from build123d import *

# Parameters (mm, degrees)
CROQUIS1_W              = 700
CROQUIS1_H              = 700
CROQUIS1_W_2            = 600
CROQUIS1_H_2            = 600
SALIENTE_EXTRUIR1_DEPTH = 50
CROQUIS2_W              = 50
CROQUIS2_H              = 50
SALIENTE_EXTRUIR2_DEPTH = 1800
CROQUIS3_W              = 700
CROQUIS3_H              = 700
CROQUIS3_W_2            = 600
CROQUIS3_H_2            = 600
SALIENTE_EXTRUIR3_DEPTH = 50
CROQUIS4_W              = 700
CROQUIS4_H              = 700
CROQUIS4_W_2            = 600
CROQUIS4_H_2            = 600
SALIENTE_EXTRUIR4_DEPTH = 50
CROQUIS6_W              = 122.530736156
CROQUIS6_H              = 155
CROQUIS6_W_2            = 72.530736156
CROQUIS6_H_2            = 80
SALIENTE_EXTRUIR5_DEPTH = 50
CROQUIS7_W              = 25
CROQUIS7_H              = 25
SALIENTE_EXTRUIR6_DEPTH = 100
SALIENTE_EXTRUIR7_DEPTH = 15


with BuildPart() as part:
    # Croquis1 → Saliente-Extruir1 (new body)
    with BuildSketch(Plane(origin=(0, 0, 0), x_dir=(1, 0, 0), z_dir=(0, 1, 0))):
        with Locations((300, 300)):
            Rectangle(CROQUIS1_W, CROQUIS1_H)
        with Locations((300, 300)):
            Rectangle(CROQUIS1_W_2, CROQUIS1_H_2, mode=Mode.SUBTRACT)
    extrude(amount=SALIENTE_EXTRUIR1_DEPTH)

    # Croquis2 → Saliente-Extruir2 (add)
    with BuildSketch(Plane.XZ):
        with Locations((625, 25)):
            Rectangle(CROQUIS2_W, CROQUIS2_H)
        with Locations((-25, 25)):
            Rectangle(CROQUIS2_W, CROQUIS2_H)
        with Locations((-25, -625)):
            Rectangle(CROQUIS2_W, CROQUIS2_H)
        with Locations((625, -625)):
            Rectangle(CROQUIS2_W, CROQUIS2_H)
    extrude(amount=SALIENTE_EXTRUIR2_DEPTH)

    # Croquis3 → Saliente-Extruir3 (add)
    with BuildSketch(Plane(origin=(0, -725, 0), x_dir=(-1, 0, 0), z_dir=(0, -1, 0))):
        with Locations((-300, 300)):
            Rectangle(CROQUIS3_W, CROQUIS3_H)
        with Locations((-300, 300)):
            Rectangle(CROQUIS3_W_2, CROQUIS3_H_2, mode=Mode.SUBTRACT)
    extrude(amount=SALIENTE_EXTRUIR3_DEPTH)

    # Croquis4 → Saliente-Extruir4 (add)
    with BuildSketch(Plane(origin=(0, -50, 0), x_dir=(-1, 0, 0), z_dir=(0, -1, 0))):
        with Locations((-300, 300)):
            Rectangle(CROQUIS4_W, CROQUIS4_H)
        with Locations((-300, 300)):
            Rectangle(CROQUIS4_W_2, CROQUIS4_H_2, mode=Mode.SUBTRACT)
    extrude(amount=SALIENTE_EXTRUIR4_DEPTH)

    # Croquis6 → Saliente-Extruir5 (add)
    with BuildSketch(Plane.XY.offset(50)):
        with Locations((446.741550776, 77.5)):
            Rectangle(CROQUIS6_W, CROQUIS6_H)
        with Locations((446.741550776, 90)):
            Rectangle(CROQUIS6_W_2, CROQUIS6_H_2, mode=Mode.SUBTRACT)
    extrude(amount=-SALIENTE_EXTRUIR5_DEPTH)

    # Croquis7 → Saliente-Extruir6 (add)
    with BuildSketch(Plane(origin=(0, 0, 0), x_dir=(-1, 0, 0), z_dir=(0, 0, -1))):
        with Locations((-445.476182698, 142.5)):
            Rectangle(CROQUIS7_W, CROQUIS7_H)
    extrude(amount=SALIENTE_EXTRUIR6_DEPTH)

    # Croquis9 → Saliente-Extruir7 (add, symmetric)
    with BuildSketch(Plane.ZY.offset(-90)):
        Polygon((0, 50), (50, 50), (50, 290), (-650, 290), (-650, 50), (-600, 50), (-600, 240), (0, 240), align=None)
    extrude(amount=SALIENTE_EXTRUIR7_DEPTH, both=True)


solid = part.part
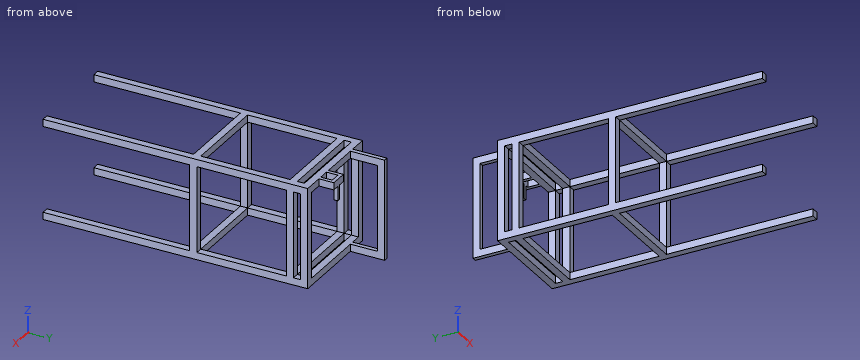
Model file for the job. Use its own axes, mm. Give positions to 0.01 mm unless a question says otherwise; leave off trailing zeros. Order: outer loops, then holes, each group sorted by start corner. A loop starts at its lowest first (then second) coordinate and runs counter-clockwise, first axis right, second up. Notation, with made-up numbers: M 43.25,30 L 75.25,30 A18 cw 75.25,44 Z; hole C -32.5,53 d8. An arc over 180 degrees is marked long. Put each result on its own line as item: value. Start each with the question number.
(1) Band-saw the part on A-A on x = 20. Give the cut face in (y, z).
(2) Drill centre lines: L1, parallel to Y at x = -13.5, z = -141; L2, parallel to Y at x = 472, z = 4; L3, parallel to X at y = -823.5, z = -608.5. Where is each one in solid material? Low to high. Write a range as [from, to].
(3) Band-saw the part on B-B on y = -300.5. Give the cut face in (x, z).
(4) Pin check, flat tips, straight feed: pin 1 Ø15 at (x, z) = (625.5, -358.5) entering from +Y; pin 2 Ø15 at (x, z) = (340.5, -631) entering from -Y. Stop position of each tip, or through.
(5) Band-saw the part on C-C on z = -259. Give the cut face in (x, y).
Results below:
1. outline: M -775,-650 L -725,-650 L -725,-600 L -775,-600 Z; M -775,0 L -725,0 L -725,50 L -775,50 Z; M -100,-650 L -50,-650 L -50,-600 L -100,-600 Z; M -100,0 L -50,0 L -50,50 L -100,50 Z; M 0,-650 L 50,-650 L 50,-600 L 0,-600 Z; M 0,0 L 50,0 L 50,50 L 0,50 Z
2. L1: y = [-775, -725], [-100, -50], [0, 50]
2. L2: y = [-775, -725], [-100, -50], [0, 50], [130, 155]
2. L3: x = [-50, 0], [600, 650]
3. outline: M -50,-650 L 0,-650 L 0,-600 L -50,-600 Z; M -50,0 L 0,0 L 0,50 L -50,50 Z; M 600,-650 L 650,-650 L 650,-600 L 600,-600 Z; M 600,0 L 650,0 L 650,50 L 600,50 Z
4. pin 1: stops at y = 50
4. pin 2: stops at y = -775
5. outline: M -50,-775 L 0,-775 L 0,-725 L -50,-725 Z; M -50,-100 L 0,-100 L 0,-50 L -50,-50 Z; M -50,0 L 0,0 L 0,50 L -50,50 Z; M 75,240 L 105,240 L 105,290 L 75,290 Z; M 600,-775 L 650,-775 L 650,-725 L 600,-725 Z; M 600,-100 L 650,-100 L 650,-50 L 600,-50 Z; M 600,0 L 650,0 L 650,50 L 600,50 Z
